Could you check a few things on this model? Use its own coordinates, in mm. A direction names the side the tool comes from. Coordinates: 2 decimals unless noted, no trailing zeros. Loops run counter-clockwise (first coordinate to the right, second up) from the corner with the lowest first, then second, coordinate; pieces in that order, holes last. Notation, with made-up numbers: (35.25, 86) -> (77.25, 86) arc R25 cw to (77.25, 99) -> close; hole circle Ø10 at (24.25, 25). An arc over 180 degrees is marked (long way). One line per question, with ' | ' between items.
from build123d import *

# Parameters (mm, degrees)
BOSS_EXTRUDE1_DEPTH = 12.5
SKETCH3_W           = 5
SKETCH3_H           = 7.5
BOSS_EXTRUDE2_DEPTH = 27.5
SKETCH4_R           = 7.5
BOSS_EXTRUDE3_DEPTH = 8
SKETCH5_W           = 10.105162594
SKETCH5_H           = 17.406531809
CUT_EXTRUDE1_DEPTH  = 151.624338723
SKETCH6_R           = 5
BOSS_EXTRUDE4_DEPTH = 6
FILLET1_R           = 10
SKETCH7_R           = 2.65
CUT_EXTRUDE2_DEPTH  = 6


with BuildPart() as part:
    # Sketch1 → Boss-Extrude1 (new, symmetric)
    with BuildSketch(Plane(origin=(0, 0, 0), x_dir=(0, 0, -1), z_dir=(1, 0, 0))):
        with BuildLine():
            Line((-19.096184677, 121.225789304), (-19.096184677, 137.404518888))
            add(Edge.make_bspline(
                [(-19.096184677, 137.404518888), (-6.467464955, 151.699126132), (18.56858261, 142.711827006)],
                knots=[0, 0, 0, 1, 1, 1], degree=2))
            add(Edge.make_bspline(
                [(18.56858261, 142.711827006), (20.515458249, 129.056565793), (17.198954708, 118.572135245)],
                knots=[0, 0, 0, 1, 1, 1], degree=2))
            add(Edge.make_bspline(
                [(17.198954708, 118.572135245), (7.355214534, 114.934231268), (-7.542469836, 112.881439696), (-19.096184677, 121.225789304)],
                knots=[0, 0, 0, 0, 1, 1, 1, 1], degree=3))
        make_face()
    extrude(amount=BOSS_EXTRUDE1_DEPTH, both=True)

    # Sketch3 → Boss-Extrude2 (add, symmetric)
    with BuildSketch(Plane(origin=(0, 0, 0), x_dir=(0, 0, -1), z_dir=(1, 0, 0))):
        with Locations((0.903815323, 129.315154096)):
            Rectangle(SKETCH3_W, SKETCH3_H)
    extrude(amount=BOSS_EXTRUDE2_DEPTH, both=True)

    # Sketch4 → Boss-Extrude3 (add)
    with BuildSketch(Plane(origin=(0, 0, -3.403815323), x_dir=(-1, 0, 0), z_dir=(0, 0, -1))):
        with Locations(Location((-21.004809472, 129.315154096, 0), (0, 0, 210))):
            Circle(SKETCH4_R)
        with Locations(Location((21.004809472, 129.315154096, 0), (0, 0, 210))):
            Circle(SKETCH4_R)
    extrude(amount=BOSS_EXTRUDE3_DEPTH)

    # Sketch5 → Cut-Extrude1 (cut, through all)
    with BuildSketch(Plane.XY.offset(-3.403815323)):
        with Locations((-26.057390769, 128.111888192)):
            Rectangle(SKETCH5_W, SKETCH5_H)
        with Locations((26.057390769, 128.111888192)):
            Rectangle(SKETCH5_W, SKETCH5_H)
    extrude(amount=CUT_EXTRUDE1_DEPTH, mode=Mode.SUBTRACT)

    # Sketch6 → Boss-Extrude4 (add)
    with BuildSketch(Plane.XY.offset(-3.403815323)):
        with Locations(Location((21.004809472, 129.315154096, 0), (0, 0, 228.590377891))):
            Circle(SKETCH6_R)
        with Locations(Location((-21.004809472, 129.315154096, 0), (0, 0, 48.590377891))):
            Circle(SKETCH6_R)
    extrude(amount=BOSS_EXTRUDE4_DEPTH)

    # Fillet1
    # the kernel refuses this fillet: 10 mm, written as the material it adds along each edge
    with BuildSketch(Plane(origin=(12.5, 125.565154096, 1.596184677), x_dir=(0, -1, 0), z_dir=(0, 0, -1)), Plane(origin=(12.5, 133.065154096, -3.403815323), x_dir=(0, 1, 0), z_dir=(0, 0, 1))) as fillet1_piece_1:
        with BuildLine():
            CenterArc((8.771382419, -10), FILLET1_R, 90, 61.299054853)
            Line((0, -5.197620333), (0, 0))
            Line((0, 0), (8.771382419, 0))
        make_face()
    extrude(amount=5)
    with BuildSketch(Plane(origin=(-12.5, 133.065154096, -3.403815323), x_dir=(0, 1, 0), z_dir=(0, 0, 1)), Plane(origin=(-12.5, 125.565154096, 1.596184677), x_dir=(0, -1, 0), z_dir=(0, 0, -1))) as fillet1_piece_2:
        with BuildLine():
            CenterArc((8.771382419, 10), FILLET1_R, 208.700945147, 61.299054853)
            Line((0, 5.197620333), (0, 0))
            Line((0, 0), (8.771382419, 0))
        make_face()
    extrude(amount=5)

    # Sketch7 → Cut-Extrude2 (cut)
    with BuildSketch(Plane.XY.offset(2.596184677)):
        with Locations((21.004809472, 129.315154096)):
            Circle(SKETCH7_R)
        with Locations((-21.004809472, 129.315154096)):
            Circle(SKETCH7_R)
    extrude(amount=-CUT_EXTRUDE2_DEPTH, mode=Mode.SUBTRACT)


with BuildPart() as part_1:
    # Body-Move/Copy1: moved
    add(part.part.moved(Location((0, -129.32, -0.9))))


solid = part_1.part
1) I need wall thicknesses on line 1 along X through (y, z) = (-5, -8); line 2 along Y through (x, z) = (-2, -1); line 3 along X through (y, z) = (-9.5, -11.5). Which ranges of each line are inside material? Lowest first, please. Write a range as from..to.
Data:
line 1: -26.6..-15.41, -12.5..12.5, 15.41..26.6 | line 2: -13.92..16.85 | line 3: -12.5..12.5
2) If we section it at A-A on x = 22.5: Please give me the cut outline in (y, z).
Data:
outline: (-7.35, -12.3) -> (7.34, -12.3) -> (7.34, -4.3) -> (4.77, -4.3) -> (4.77, 1.7) -> (2.18, 1.7) -> (2.18, -4.3) -> (-2.19, -4.3) -> (-2.19, 1.7) -> (-4.78, 1.7) -> (-4.78, -4.3) -> (-7.35, -4.3) -> close
3) I'm going to push flat-ended pins straight in: pin 1 Ø2 at (x, z) = (3.5, 5.5) entering from -Y; pin 2 Ø3 at (y, z) = (13.5, 1.5) entering from +X; pin 3 Ø8 at (y, z) = (-2.5, 3.5) entering from +X. Where does each tip first touch, or does it pass through?
Data:
pin 1: y = -13.52 | pin 2: x = 12.5 | pin 3: x = 26
4) We'd pull the mould along Y, two halves only. Please class faces 6 (the face through (19.052, 1.786, -1.262)), 7 (the face through (-12.5, 3, 3)), 8 (the face through (21, 0, -4.304)), 9 (the face through (13.86, -7.49, -1.77)): pulls with the +Y half, pulls with the -Y half, needs draft (parallel to the pull), parting line crosses it, or undercut.
Data:
face 6: undercut | face 7: needs draft | face 8: undercut | face 9: pulls with the -Y half
5) On a 3-axis mill with a long thin cutter (end or side, diameter ignored), from which of +Z, -Z, +X, -X, +Y, -Y can I reach the whole of each face in a straight line? I mean faces 1 (the face through (-18, 0, 1.696)), 2 (the face through (13, 0, -4.304)), 3 (the face through (18, 0, 1.696)), 4 (the face through (13.86, 7.48, -1.84)), 5 (the face through (25.977, 0.524, -1.346)). Say none if no direction works.
Data:
face 1: +Z, -X, +Y, -Y | face 2: -Z | face 3: +Z, +X, +Y, -Y | face 4: +Z, +Y | face 5: +Z
6) If we section it at B-B on z = -10: Give the number of separate pieces and of enclosed holes in the cut face, and give its area (3 significant figures).
Data:
separate pieces: 3 | enclosed holes: 0 | area: 1,080 mm²
7) If we section it at C-C on x = -19.5: Please give me the cut outline in (y, z).
Data:
outline: (-7.35, -12.3) -> (7.34, -12.3) -> (7.34, -4.3) -> (4.76, -4.3) -> (4.76, 1.7) -> (2.18, 1.7) -> (2.18, -4.3) -> (-2.19, -4.3) -> (-2.19, 1.7) -> (-4.77, 1.7) -> (-4.77, -4.3) -> (-7.35, -4.3) -> close
